Input: part model. Units: mm. Frame: model coordinates. Give positions to 0.01 mm unless a question says otherwise; leave off trailing zeros. Order: outer loops, then holes, each group sorted by start corner. A loop starts at its lowest first (then second) coordinate and runs counter-clockwise, first axis right, second up. Notation, with made-up numbers: (-2.5, 69) - (52.5, 69) arc R18 ccw to (52.5, 78) - close; hole circle Ø6 at (-28.5, 29). An arc over 180 degrees is marked (long way). Answer in a Markdown table with one row per item. Add a question column.
from build123d import *

# Parameters (mm, degrees)
SKETCH4_W               = 80
SKETCH4_H               = 100
CUT_EXTRUDE1_DEPTH      = 200
CUT_EXTRUDE1_DEPTH_BACK = 200
SKETCH5_R               = 10
BOSS_EXTRUDE1_DEPTH     = 60
SKETCH6_R               = 10
BOSS_EXTRUDE2_DEPTH     = 80
CUT_EXTRUDE2_DEPTH      = 64.245553203
CUT_EXTRUDE2_DEPTH_BACK = 64.245553203


with BuildPart() as part:
    # Sketch3 → Revolve1 (revolve)
    with BuildSketch(Plane.XY):
        with BuildLine():
            Line((0, 70), (0, -70))
            ThreePointArc((0, -70), (70, 0), (0, 70))
        make_face()
    revolve(axis=Axis((0, 136.094420601, 0), (0, -1, 0)))

    # Sketch4 → Cut-Extrude1 (cut, two sides)
    with BuildSketch(Plane(origin=(0, 0, 0), x_dir=(1, 0, 0), z_dir=(0, 1, 0))) as cut_extrude1_sk:
        with Locations((0, -20)):
            Rectangle(SKETCH4_W, SKETCH4_H)
    extrude(amount=CUT_EXTRUDE1_DEPTH, mode=Mode.SUBTRACT)
    extrude(cut_extrude1_sk.sketch, amount=-CUT_EXTRUDE1_DEPTH_BACK, mode=Mode.SUBTRACT)

    # Sketch5 → Boss-Extrude1 (add)
    with BuildSketch(Plane.XY.offset(-30)):
        Circle(SKETCH5_R)
    extrude(amount=-BOSS_EXTRUDE1_DEPTH)

    # Sketch6 → Boss-Extrude2 (add)
    with BuildSketch(Plane(origin=(-40, 0, 0), x_dir=(0, 0, -1), z_dir=(1, 0, 0))):
        Circle(SKETCH6_R)
    extrude(amount=BOSS_EXTRUDE2_DEPTH)

    # Sketch7 → Cut-Extrude2 (cut, two sides)
    with BuildSketch(Plane(origin=(0, 0, 0), x_dir=(1, 0, 0), z_dir=(0, 1, 0))) as cut_extrude2_sk:
        with BuildLine():
            Line((40, 30), (-40, 30))
            ThreePointArc((-40, 30), (0, 46.568542495), (40, 30))
        make_face()
    extrude(amount=CUT_EXTRUDE2_DEPTH, mode=Mode.SUBTRACT)
    extrude(cut_extrude2_sk.sketch, amount=-CUT_EXTRUDE2_DEPTH_BACK, mode=Mode.SUBTRACT)


solid = part.part
Q1. Section A-A, the plane x = 6.5. Return loops of the section in (y, z), then the cut area to 3 significant figures.
Q2. Pull-direction query (X, two-part tool) for faces 1 (the flat face through (40, -1, 14)), 2 (the cylindrical face through (-2.17, -9.76, -79.5)), 3 (the flat face through (0, 0, -90)); classes: +X half, -X half, draft (parallel to the pull), parting line (faces both ways), or undercut.
Q3. Contact query for flat-ended pins moving along their axis: P1, Ø5, axis at x = -26.5, y = 32, coming from the +Z side; P2, Ø2, axis at x = 0.5, z = 3, coming from the +Y side; P3, Ø10, axis at x = 48.5, z = 36, coming from the +Y side. Output: stop coordinate, or through.
Q4. Section B-B, the plane z = 0. Return loops of the section in (x, y).
Q5. Section C-C, the plane y = 0. Return loops of the section in (x, z).
Q6. Section D-D, the plane z = 30.5. Return loops of the section in (x, y).
Q7. Line query: probe 1 along X at (y, z) = (5, 23.5); probe 2 along X at (y, z) = (42, 30.5); probe 3 along Z at (x, y) = (4.5, 4). Output: solid intervals per line, ascending.
Computed:
| question | item | result |
|---|---|---|
| 1 | outline | (-52.19, -46.19) arc R69.7 ccw to (-7.6, -69.28) - (-7.6, -90) - (7.6, -90) - (7.6, -69.28) arc R69.7 ccw to (52.19, -46.19) - close; circle Ø20 at (0, 0) |
| 1 | area | 2,320 mm^2 |
| 2 | face 1 | undercut |
| 2 | face 2 | parting line |
| 2 | face 3 | draft |
| 3 | P1 | stops at z = -38.57 |
| 3 | P2 | stops at y = 9.8 |
| 3 | P3 | stops at y = 42.79 |
| 4 | outline | (-40, -57.45) - (-40, -10) - (40, -10) - (40, -57.45) arc R70 ccw to (40, 57.45) - (40, 10) - (-40, 10) - (-40, 57.45) arc R70 ccw to start |
| 5 | outline | (-40, 10) - (-40, 57.45) arc R70 ccw to (-10, -69.28) - (-10, -90) - (10, -90) - (10, -69.28) arc R70 ccw to (40, 57.45) - (40, 10) - close; hole (-40, -30) arc R56.57 ccw to (40, -30) - (40, -10) - (-40, -10) - close |
| 6 | outline | (-40, -48.68) - (-40, 48.68) arc R63.01 ccw to start; (40, -48.68) arc R63.01 ccw to (40, 48.68) - close |
| 7 | probe 1 | x = -65.75 to -40, 40 to 65.75 |
| 7 | probe 2 | x = -46.97 to -40, 40 to 46.97 |
| 7 | probe 3 | z = -90 to -46.39, -9.17 to 9.17 |
